Could you check a few things on this model? Use its own coordinates, in mm. Round coordinates to 2 decimals unless told otherwise and drop trailing zeros. Write each loop counter-clockwise with the first axis right and the second up, starting at its lowest first coordinate (ties: lowest second). Pieces come first, ordered by that corner, then holes. Notation, with made-up numbers: (-14.75, 19) -> (1.25, 19) arc R19 cw to (1.25, 41) -> close; hole circle Ø3 at (70, 47). An arc over 180 degrees is marked (long way). Answer in a Markdown table with one row per item.
from build123d import *

# Parameters (mm, degrees)
SKETCH_2_W             = 38
SKETCH_2_H             = 39
EXTRUDE_1_DEPTH        = 2
CHAMFER_3_SIZE         = 1
SKETCH_7_R             = 4.25
CUT_EXTRUDE_3_DEPTH    = 10
SKETCH_8_W             = 2
SKETCH_8_H             = 39
CUT_EXTRUDE_4_DEPTH    = 10
FILLET_3_R             = 2
SKETCH_9_R             = 2
EXTRUDE_1_2_DEPTH      = 21
SKETCH_10_W            = 3
SKETCH_10_H            = 39
CUT_EXTRUDE_1_DEPTH    = 10
FILLET_5_R             = 2
CHAMFER_5_SIZE         = 0.5
HOLE_WIZARD_M2_5_3_D   = 2.05
HOLE_WIZARD_M2_1_D     = 1.6
HOLE_WIZARD_M2_1_DEPTH = 7
HOLE_WIZARD_M2_1_TIP   = 0.480688495
CUT_EXTRUDE_2_DEPTH    = 10
SKETCH_24_W            = 71.290640242
SKETCH_24_H            = 51.144653494
CUT_EXTRUDE_3_2_DEPTH  = 10
SKETCH_25_R            = 6.539265834
CUT_EXTRUDE_4_2_DEPTH  = 32
HOLE_WIZARD_M2_2_D     = 1.6
HOLE_WIZARD_M2_2_DEPTH = 7
HOLE_WIZARD_M2_2_TIP   = 0.480688495
FILLET_6_SIZE          = 0.5


with BuildPart() as part:
    # 草图2 → Extrude 1 (new body)
    with BuildSketch(Plane.XY):
        Rectangle(SKETCH_2_W, SKETCH_2_H)
    extrude(amount=EXTRUDE_1_DEPTH)

    # 倒角3
    chamfer_3_edges = [part.edges().sort_by_distance(p)[0] for p in [
        (-19, 19.5, 1),
        (-19, -19.5, 1),
    ]]
    chamfer(chamfer_3_edges, length=CHAMFER_3_SIZE)

    # 草图7 → Cut-Extrude 3 (cut)
    with BuildSketch(Plane.XY.offset(2)):
        with Locations((2, 0)):
            Circle(SKETCH_7_R)
    extrude(amount=-CUT_EXTRUDE_3_DEPTH, mode=Mode.SUBTRACT)

    # 草图8 → Cut-Extrude 4 (cut)
    with BuildSketch(Plane.XY.offset(2)):
        with Locations((-18, 0)):
            Rectangle(SKETCH_8_W, SKETCH_8_H)
    extrude(amount=-CUT_EXTRUDE_4_DEPTH, mode=Mode.SUBTRACT)

    # 圆角3
    fillet_3_edges = [part.edges().sort_by_distance(p)[0] for p in [
        (-17, 19.5, 1),
        (-17, -19.5, 1),
    ]]
    fillet(fillet_3_edges, radius=FILLET_3_R)

    # 草图9 → Extrude 1 2 (add)
    with BuildSketch(Plane.XY.offset(2)):
        with Locations((-15, 17.5)):
            Circle(SKETCH_9_R)
        with Locations((-15, -17.5)):
            Circle(SKETCH_9_R)
    extrude_1_2 = extrude(amount=EXTRUDE_1_2_DEPTH)

    # 镜向1: Extrude 1 2 across plane
    add(extrude_1_2.mirror(Plane.ZX))

    # 草图10 → 切除-拉伸1 (cut)
    with BuildSketch(Plane(origin=(0, 0, 0), x_dir=(-1, 0, 0), z_dir=(0, 0, -1))):
        with Locations((-17.5, 0)):
            Rectangle(SKETCH_10_W, SKETCH_10_H)
    extrude(amount=-CUT_EXTRUDE_1_DEPTH, mode=Mode.SUBTRACT)

    # 圆角5
    fillet_5_edges = [part.edges().sort_by_distance(p)[0] for p in [
        (16, -19.5, 1),
        (16, 19.5, 1),
    ]]
    fillet(fillet_5_edges, radius=FILLET_5_R)

    # 倒角5
    chamfer_5_edges = [part.edges().sort_by_distance(p)[0] for p in [
        (-17, -17.5, 23),
        (-17, 17.5, 23),
        (15.414213562, 18.914213562, 0),
        (16, 0, 0),
        (-0.5, 19.5, 0),
        (15.414213562, -18.914213562, 0),
        (-16.414213562, 18.914213562, 0),
        (-0.5, -19.5, 0),
        (-17, 0, 0),
        (-16.414213562, -18.914213562, 0),
    ]]
    chamfer(chamfer_5_edges, length=CHAMFER_5_SIZE)

    # M2.5 螺纹孔3 (through all)
    with Locations(Plane(origin=(9.5, 15.5, 0), x_dir=(-1, 0, 0), z_dir=(0, 0, -1))):
        with Locations((0, 0), (15, 0), (0, -31), (15, -31)):
            Hole(HOLE_WIZARD_M2_5_3_D / 2)

    # M2 螺纹孔1
    with Locations(Plane(origin=(-15, 17.5, 23), x_dir=(1, 0, 0), z_dir=(0, 0, 1))):
        with Locations((0, 0), (0, -35)):
            Hole(HOLE_WIZARD_M2_1_D / 2, depth=HOLE_WIZARD_M2_1_DEPTH)
            with Locations((0, 0, -(HOLE_WIZARD_M2_1_DEPTH + HOLE_WIZARD_M2_1_TIP / 2))):  # 118° drill point
                Cone(0, HOLE_WIZARD_M2_1_D / 2, HOLE_WIZARD_M2_1_TIP, mode=Mode.SUBTRACT)

    # 草图23 → 切除-拉伸2 (cut)
    with BuildSketch(Plane(origin=(0, 0, 0), x_dir=(-1, 0, 0), z_dir=(0, 0, -1))):
        with BuildLine():
            Line((-0.95, 16.2), (-0.95, 9.8))
            ThreePointArc((-0.95, 9.8), (-2, 8.75), (-3.05, 9.8))
            Line((-3.05, 9.8), (-3.05, 16.2))
            ThreePointArc((-3.05, 16.2), (-2, 17.25), (-0.95, 16.2))
        make_face()
    cut_extrude_2 = extrude(amount=-CUT_EXTRUDE_2_DEPTH, mode=Mode.SUBTRACT)

    # 镜向2: 切除-拉伸2 across plane
    add(cut_extrude_2.mirror(Plane.ZX), mode=Mode.SUBTRACT)

    # 草图24 → Cut-Extrude 3 2 (cut)
    with BuildSketch(Plane.XY.offset(2)):
        Rectangle(SKETCH_24_W, SKETCH_24_H)
    extrude(amount=-CUT_EXTRUDE_3_2_DEPTH, mode=Mode.SUBTRACT)


with BuildPart() as cut_extrude_3_2_piece_1:
    # of the separate pieces the step leaves, piece 1, a body of its own (cut_extrude_3_2_pieces)
    add(part.part.solids().sort_by_distance((-13, 17.5, 22.5))[0])

    # 草图25 → Cut-Extrude 4 2 (cut)
    with BuildSketch(Plane(origin=(0, 0, 2), x_dir=(-1, 0, 0), z_dir=(0, 0, -1))):
        with Locations((15, 17.5)):
            Circle(SKETCH_25_R)
    extrude(amount=-CUT_EXTRUDE_4_2_DEPTH, mode=Mode.SUBTRACT)


with BuildPart() as cut_extrude_3_2_piece_2:
    # of the separate pieces the step leaves, piece 2, a body of its own (cut_extrude_3_2_pieces)
    add(part.part.solids().sort_by_distance((-13, -17.5, 2))[0])

    # M2 螺纹孔2
    with Locations(Plane(origin=(-15, -17.5, 2), x_dir=(-1, 0, 0), z_dir=(0, 0, -1))):
        with Locations((0, 0)):
            Hole(HOLE_WIZARD_M2_2_D / 2, depth=HOLE_WIZARD_M2_2_DEPTH)
            with Locations((0, 0, -(HOLE_WIZARD_M2_2_DEPTH + HOLE_WIZARD_M2_2_TIP / 2))):  # 118° drill point
                Cone(0, HOLE_WIZARD_M2_2_D / 2, HOLE_WIZARD_M2_2_TIP, mode=Mode.SUBTRACT)

    # 圆角6
    # a fillet whose section is not a circle: 0.5 mm, written as the material it takes off along each edge
    with BuildSketch(Plane(origin=(-15, -17.5, 2), x_dir=(1, 0, 0), z_dir=(0, -1, 0))) as fillet_6_piece_1:
        with BuildLine():
            Bezier((2, FILLET_6_SIZE), (2, 0), (2 - FILLET_6_SIZE, 0), weights=[1, 0.035355339, 1])
            Line((2 - FILLET_6_SIZE, 0), (2, 0))
            Line((2, 0), (2, FILLET_6_SIZE))
        make_face()
    revolve(axis=Axis((-15, -17.5, 2), (0, 0, 1)), mode=Mode.SUBTRACT)


solid = cut_extrude_3_2_piece_2.part
1) Imagine slicing it at B-B, the plane z = 10.5. Please give me the cut outline in (x, y), plus the area to 3 significant figures.
Findings:
| item | result |
|---|---|
| outline | circle Ø4 at (-15, -17.5) |
| area | 12.6 mm^2 |
2) For pin 1 (2 mm diameter, centred on x = -14.5, z = 15, fed in from -Y); pin 2 (1.5 mm diameter, centred on x = -15, y = -17.5, fed in from +Z); pin 3 (1.3 mm diameter, centred on x = -15, y = -17.5, fed in from -Z); pin 4 (1.3 mm diameter, centred on x = -15, y = -17.5, fed in from +Z), each with a flat end and sliding along its axis, tell me the tip position at first contact or that it passes through.
Findings:
| item | result |
|---|---|
| pin 1 | stops at y = -19.5 |
| pin 2 | stops at z = 15.97 |
| pin 3 | stops at z = 9.09 |
| pin 4 | stops at z = 15.91 |
3) Thinking about a two-plate mould opening in Y: for faces 1 (the face through (-14, -18, 2)), 2 (the face through (-15.63, -17.99, 5.55)), 3 (the face through (-14.37, -17.99, 19.45)), 4 (the face through (-15.26, -15.517, 12.36)), which applies, +Y half, -Y half, draft (parallel to the pull), parting line (faces both ways), or undercut?
Findings:
| item | result |
|---|---|
| face 1 | draft |
| face 2 | undercut |
| face 3 | undercut |
| face 4 | parting line |
4) Please list where these lines run through material, in increasing order: line 1 (Y direction, x = -15, z = 7.75); line 2 (X direction, y = -17.85, z = 18.5); line 3 (X direction, y = -17.95, z = 21).
Findings:
| item | result |
|---|---|
| line 1 | y = -19.5 to -18.3, -16.7 to -15.5 |
| line 2 | x = -16.97 to -15.72, -14.28 to -13.03 |
| line 3 | x = -16.95 to -15.66, -14.34 to -13.05 |
5) Imagine slicing it at A-A, the plane z = 8.25. Please give me the cut outline in (x, y), plus the area to 3 significant figures.
Findings:
| item | result |
|---|---|
| outline | circle Ø4 at (-15, -17.5); hole circle Ø1.6 at (-15, -17.5) |
| area | 10.6 mm^2 |
